Design review of the part built by this model. Coordinates are the model's own, in mm. A direction names the side the tool comes from. Coordinates: 2 decimals unless noted, no trailing zeros. Write each loop counter-clockwise with the first axis right and the second up, starting at its lowest first coordinate (ties: lowest second). Pieces come first, ordered by that corner, then holes.
Q1. Insertion check: pin 1 (1.9 mm diameter, centred on x = -1.5, y = -48, fed in from -Z); pin 2 (1.5 mm diameter, centred on x = 2.5, z = -92.5, fed in from -Y). Each pin has a flat end and moves straight along its axis. Give the tip position at first contact, or say it passes through.
Q2. Mouldability with a two-part tool opening along Y and no side actions: class faces 1 (the flat face through (3.175, 38.4, -72)), 2 (the flat face through (0, 53.975, -74.9)), 3 (the flat face through (0, -38.1, -29)) as pulls with the +Y half, pulls with the -Y half, needs draft (parallel to the pull), parting line crosses it, or undercut.
Q3. For probe 1 along X at (y, z) = (50, -215.9) (3 decimals); probe 2 along Y at (x, z) = (-1.25, -5); probe 3 along Z at (x, y) = (0, 49.5), list the stretches that pass through material, from the lowest coordinate up.
Q4. Machinability: for faces 4 (the flat face through (0, 38.1, -122)), 5 (the flat face through (0, -57.15, -28)), 6 (the flat face through (0, 57.15, -35)), 7 (the flat face through (0, -48, -57.15)), 8 (the flat face through (0, 53.975, -217.4)), which of the approach directions +Z, -Z, +X, -X, +Y, -Y give a long, thin tool a straight path to every point of the face, cutting with its end or side? Answer none if there is none.
Q5. Take a section at A-A (z = -166). Give the boundary of the cut face in (x, y) (3 decimals), and give its area (3 significant figures).
```python
from build123d import *

# Parameters (mm, degrees)
SKETCH1_R                 = 3.175
BOSS_EXTRUDE1_DEPTH       = 3.175
F_4_40_TAPPED_HOLE1_D     = 2.2606
F_4_40_TAPPED_HOLE1_DEPTH = 7.62
F_4_40_TAPPED_HOLE1_TIP   = 0.679152758


with BuildPart() as part:
    # Sketch1 → Boss-Extrude1 (new body, symmetric)
    with BuildSketch(Plane(origin=(0, 0, 0), x_dir=(0, 0, -1), z_dir=(1, 0, 0))):
        with BuildLine():
            Line((57.15, -38.1), (0, -38.1))
            ThreePointArc((0, -38.1), (-38.1, 0), (0, 38.1))
            Line((0, 38.1), (247.65, 38.1))
            Line((247.65, 38.1), (247.65, 57.15))
            Line((247.65, 57.15), (222.25, 57.15))
            Line((222.25, 57.15), (222.25, 53.975))
            Line((222.25, 53.975), (209.55, 53.975))
            Line((209.55, 53.975), (209.55, 57.15))
            Line((209.55, 57.15), (82.55, 57.15))
            Line((82.55, 57.15), (82.55, 53.975))
            Line((82.55, 53.975), (69.85, 53.975))
            Line((69.85, 53.975), (69.85, 57.15))
            Line((69.85, 57.15), (0, 57.15))
            ThreePointArc((0, 57.15), (-57.15, 0), (0, -57.15))
            Line((0, -57.15), (57.15, -57.15))
            Line((57.15, -57.15), (57.15, -38.1))
        make_face()
        with Locations((238.125, 47.625)):
            Circle(SKETCH1_R, mode=Mode.SUBTRACT)
    extrude(amount=BOSS_EXTRUDE1_DEPTH, both=True)

    # #4-40 Tapped Hole1
    with Locations(Plane(origin=(0, 53.975, 0), x_dir=(1, 0, 0), z_dir=(0, 1, 0))):
        with Locations((0, 76.2), (0, 215.9)):
            Hole(F_4_40_TAPPED_HOLE1_D / 2, depth=F_4_40_TAPPED_HOLE1_DEPTH)
            with Locations((0, 0, -(F_4_40_TAPPED_HOLE1_DEPTH + F_4_40_TAPPED_HOLE1_TIP / 2))):  # 118° drill point
                Cone(0, F_4_40_TAPPED_HOLE1_D / 2, F_4_40_TAPPED_HOLE1_TIP, mode=Mode.SUBTRACT)


solid = part.part
```
Response:
1. pin 1: stops at z = -57.15
1. pin 2: stops at y = 38.1
2. face 1: needs draft
2. face 2: pulls with the +Y half
2. face 3: undercut
3. probe 1: x = -3.175 to -1.13, 1.13 to 3.175
3. probe 2: y = -57.15 to -38.1, 38.1 to 57.15
3. probe 3: z = -247.65 to -240.69, -235.56 to -217.03, -214.77 to -77.33, -75.07 to 28.56
4. face 4: -Z, +X, -X
4. face 5: +Z, -Z, +X, -X, -Y
4. face 6: +Z, -Z, +X, -X, +Y
4. face 7: -Z, +X, -X, -Y
4. face 8: +X, -X, +Y
5. outline: (-3.175, 38.1) - (3.175, 38.1) - (3.175, 57.15) - (-3.175, 57.15) - close
5. area: 121 mm2
